from build123d import *

# Parameters (mm, degrees)
SKETCH_1_R           = 14.375
EXTRUDE_1_DEPTH      = 10
EXTRUDE_1_DEPTH_BACK = 10
EXTRUDE_2_DEPTH      = 20
SKETCH_10_R          = 4
CUT_EXTRUDE_1_DEPTH  = 21
SKETCH_11_R          = 5
CUT_EXTRUDE_2_DEPTH  = 4
SKETCH_12_R          = 5
CUT_EXTRUDE_3_DEPTH  = 4


with BuildPart() as part:
    # 草图1 → 凸台-拉伸1 (new body, two sides)
    with BuildSketch(Plane.XY) as extrude_1_sk:
        Circle(SKETCH_1_R)
    extrude(amount=EXTRUDE_1_DEPTH)
    extrude(extrude_1_sk.sketch, amount=-EXTRUDE_1_DEPTH_BACK)

    # 草图2 → 凸台-拉伸2 (add)
    with BuildSketch(Plane.XY.offset(10)):
        with BuildLine():
            Line((-15, 42.426406871), (-15, 14.98697351))
            ThreePointArc((-15, 14.98697351), (-3.991720171, 10.825317547), (0.625, 0))
            Line((0.625, 0), (15, 0))
            ThreePointArc((15, 0), (6.742346142, 25.980762114), (-15, 42.426406871))
        make_face()
    extrude(amount=-EXTRUDE_2_DEPTH)

    # 草图10 → 切除-拉伸1 (cut, through all)
    with BuildSketch(Plane.XY.offset(10)):
        Circle(SKETCH_10_R)
    extrude(amount=-CUT_EXTRUDE_1_DEPTH, mode=Mode.SUBTRACT)

    # 草图11 → 切除-拉伸2 (cut)
    with BuildSketch(Plane(origin=(0, 0, -10), x_dir=(-1, 0, 0), z_dir=(0, 0, -1))):
        Circle(SKETCH_11_R)
    extrude(amount=-CUT_EXTRUDE_2_DEPTH, mode=Mode.SUBTRACT)

    # 草图12 → 切除-拉伸3 (cut)
    with BuildSketch(Plane.XY.offset(10)):
        Circle(SKETCH_12_R)
    extrude(amount=-CUT_EXTRUDE_3_DEPTH, mode=Mode.SUBTRACT)


solid = part.part
Design review of the part built by this model. Coordinates are the model's own, in mm. A direction names the side the tool comes from. Round coordinates to 2 decimals unless told otherwise and drop trailing zeros. Write each loop counter-clockwise with the first axis right and the second up, starting at its lowest first coordinate (ties: lowest second). Pieces come first, ordered by that corner, then holes. Notation, with made-up numbers: (82.25, 18) - (92.25, 18) arc R32 ccw to (92.25, 57) - close; hole circle Ø2 at (-30.5, -9). An arc over 180 degrees is marked (long way). Use a Markdown table: item, result. Add a question column.
1. Wall thickness on probe 1 along Y at (x, z) = (-11, 4); probe 2 along X at (y, z) = (16, -5.75); probe 3 along Y at (x, z) = (1, 8.75): over which ranges is each line inside the solid? List them lowest first.
2. We need section C-C (z = 4). State the section outline as (x, y) points (3 decimals).
3. We need section B-B (x = 0). State the section outline as (y, z) points (3 decimals).
4. For faces 1 (the face through (-1.08, -4.88, 8.03)), 2 (the face through (-0.867, -3.905, 0.084)), 3 (the face through (1.08, -4.88, -8.03)), list the 3-axis set-ups (+Z, -Z, +X, -X, +Y, -Y) from which the entire face can be reached by the end or side of a thin tool; tool diameter is ignored.
5. Clearance check with flat-ended pins moving along their axes: pin 1 (9 mm diameter, centred on x = 0, y = 0, fed in from -Z); pin 2 (10 mm diameter, centred on x = -9, z = 1.5, fed in from -Y); pin 3 (2 mm diameter, centred on x = -10.5, z = -4.5, fed in from -Y); pin 4 (16 mm diameter, centred on x = 0, y = 0, fed in from -Z). State where each tip first meets the part, or that it passes through.
6. We need section D-D (z = -6.75). State the section outline as (x, y) points (3 decimals).
7. We need section A-A (y = 1.5). State the section outline as (x, z) points (3 decimals), then the cut area to 3 significant figures.
Output:
| question | item | result |
|---|---|---|
| 1 | probe 1 | y = -9.25 to 9.25, 14.62 to 40.79 |
| 1 | probe 2 | x = -15 to 12.06 |
| 1 | probe 3 | y = -14.34 to -4.9, 4.9 to 32.62 |
| 2 | outline | (-15, 14.987) arc R15 cw to (-6.549, 12.797) arc R14.375 ccw (long way) to (14.375, 0) - (15, 0) arc R45 ccw to (-15, 42.426) - close; hole circle Ø8 at (0, 0) |
| 3 | outline | (-14.375, -10) - (-5, -10) - (-5, -6) - (-4, -6) - (-4, 6) - (-5, 6) - (-5, 10) - (-14.375, 10) - close; (4, -6) - (5, -6) - (5, -10) - (33.541, -10) - (33.541, 10) - (5, 10) - (5, 6) - (4, 6) - close |
| 4 | face 1 | +Z |
| 4 | face 2 | +Z, -Z |
| 4 | face 3 | -Z |
| 5 | pin 1 | stops at z = -6 |
| 5 | pin 2 | stops at y = -13.81 |
| 5 | pin 3 | stops at y = -10.79 |
| 5 | pin 4 | stops at z = -10 |
| 6 | outline | (-15, 14.987) arc R15 cw to (-6.549, 12.797) arc R14.375 ccw (long way) to (14.375, 0) - (15, 0) arc R45 ccw to (-15, 42.426) - close; hole circle Ø10 at (0, 0) |
| 7 | outline | (-14.297, -10) - (-4.77, -10) - (-4.77, -6) - (-3.708, -6) - (-3.708, 6) - (-4.77, 6) - (-4.77, 10) - (-14.297, 10) - close; (3.708, -6) - (4.77, -6) - (4.77, -10) - (14.975, -10) - (14.975, 10) - (4.77, 10) - (4.77, 6) - (3.708, 6) - close |
| 7 | area | 420 mm2 |
